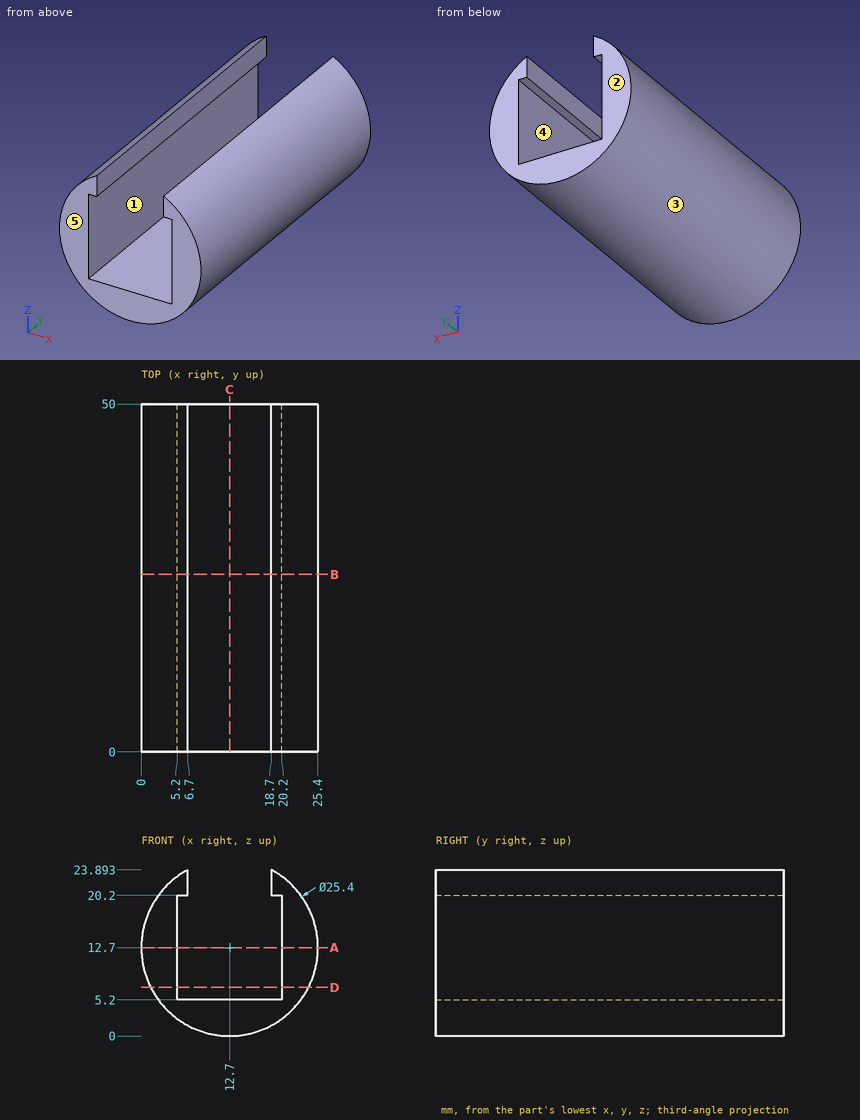
Can you work these out from the drawing? Everything is in mm from the part's minimum corner. A direction names the side the tool comes from. Round coordinates to 2 decimals unless told otherwise and drop trailing zeros. Write each loop counter-clockwise with the first axis right and the second up, starting at its lowest first coordinate (ties: lowest second). Pieces come first, ordered by that corner, then holes.
1. I need wall thicknesses on L1, parallel to X at y = 16, z = 12.75; L2, parallel to X at y = 35.5, z = 11.25; L3, parallel to Z at x = 6.5, y = 16 (1 decimal). Which ranges of each line are inside material? Lowest first, please.
2. For the marked faces 1 and 2, which set-ups out of +Z, -Z, +X, -X, +Y, -Y let a thin tool reach every point of the face, with its end or its side?
3. Suppose I cut it at B-B (y = 25.5). List the corners of the cut face in (x, z) for me, and give its area (3 significant figures).
4. If we mould it in two halves opening along Z, with no side actions, what happens to the marked faces 3, 4 and 5? For each: released by +Z, released by -Z, zero draft, split by the parting line, or undercut.
5. Will these pins go through, and if not, where does the flat tip stop? pin 1 Ø2 at (x, z) = (8.5, 19.5) entering from +Y; pin 2 Ø1.7 at (x, y) = (5.5, 31) entering from -Z; pin 3 Ø0.5 at (x, y) = (19.5, 14) entering from -Z; pin 4 Ø3 at (y, z) = (26.5, 22.5) entering from -X.
6. Suppose I cut it at A-A (z = 12.7). List the corners of the cut face in (x, y) for me.
7. Suppose I cut it at D-D (z = 7). List the corners of the cut face in (x, y) for me, and give its area (3 significant figures).
8. Suppose I cut it at C-C (x = 12.7). List the corners of the cut face in (y, z) for me, and give its area (3 significant figures).
Answer sheet:
1. L1: x = 0 to 5.2, 20.2 to 25.4
1. L2: x = 0.08 to 5.2, 20.2 to 25.32
1. L3: z = 1.6 to 5.2, 20.2 to 23.8
2. face 1: +Y, -Y
2. face 2: +Z, -Z, +X, -X, +Y
3. outline: (5.2, 5.2) - (5.2, 20.2) - (6.7, 20.2) - (6.7, 23.89) arc R12.7 ccw (long way) to (18.7, 23.89) - (18.7, 20.2) - (20.2, 20.2) - (20.2, 5.2) - close
3. area: 225 mm2
4. face 3: split by the parting line
4. face 4: undercut
4. face 5: zero draft
5. pin 1: passes through
5. pin 2: stops at z = 1.7
5. pin 3: stops at z = 1.82
5. pin 4: stops at x = 3.09
6. outline: (0, 0) - (5.2, 0) - (5.2, 50) - (0, 50) - close; (20.2, 0) - (25.4, 0) - (25.4, 50) - (20.2, 50) - close
7. outline: (1.35, 0) - (5.2, 0) - (5.2, 50) - (1.35, 50) - close; (20.2, 0) - (24.05, 0) - (24.05, 50) - (20.2, 50) - close
7. area: 385 mm2
8. outline: (0, 0) - (50, 0) - (50, 5.2) - (0, 5.2) - close
8. area: 260 mm2
